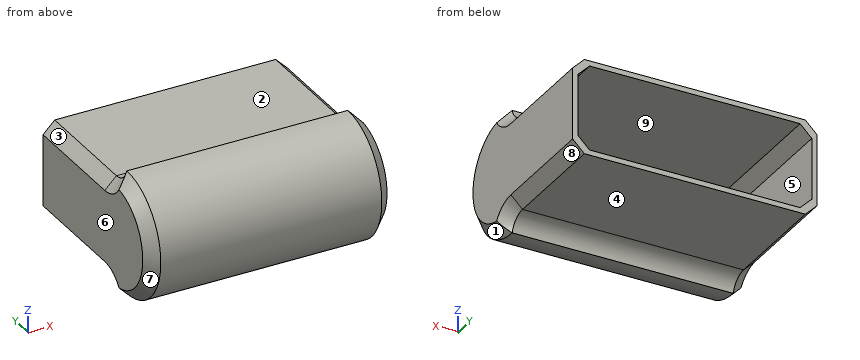
from build123d import *

# Parameters (mm, degrees)
F4_DEPTH      = 0.8
F4_DEPTH_BACK = 36.9
F5_DEPTH      = 36.1
F6_T1_DEPTH   = 37.7
F7_SIZE       = 1.8
F8_SIZE       = 1.8


# Not quite as in the source:
# - a fillet or chamfer that OpenCascade refuses, or shapes differently, is made with other operations: its cross-section is extruded or revolved along the edge and cut away or added


with BuildPart() as f4:
    # F3 (on Right) → F4 (new body, two sides)
    with BuildSketch(Plane.YZ) as f4_sk:
        with BuildLine():
            Line((20.2, 6.5358882766), (0, 6.5358882766))
            ThreePointArc((0, 6.5358882766), (-6.5358882766, 0), (0, -6.5358882766))
            Line((0, -6.5358882766), (20.2, -6.5358882766))
            Line((20.2, -6.5358882766), (20.2, 6.5358882766))
        make_face()
        with BuildLine():
            ThreePointArc((0, -6.5358882766), (-6.5358882766, 0), (0, 6.5358882766))
            Line((0, 6.5358882766), (20.2, 6.5358882766))
            Line((20.2, 6.5358882766), (20.2, 7.3358882766))
            Line((20.2, 7.3358882766), (0, 7.3358882766))
            Line((0, 7.3358882766), (0, 9.5358882766))
            ThreePointArc((0, 9.5358882766), (-9.5358882766, 0), (0, -9.5358882766))
            Line((0, -9.5358882766), (0, -7.3358882766))
            Line((0, -7.3358882766), (20.2, -7.3358882766))
            Line((20.2, -7.3358882766), (20.2, -6.5358882766))
            Line((20.2, -6.5358882766), (0, -6.5358882766))
        make_face()
    extrude(amount=-F4_DEPTH)
    extrude(f4_sk.sketch, amount=F4_DEPTH_BACK)

    # F3 (on Right) → F5 (cut)
    with BuildSketch(Plane.YZ):
        with BuildLine():
            Line((20.2, 6.5358882766), (0, 6.5358882766))
            ThreePointArc((0, 6.5358882766), (-6.5358882766, 0), (0, -6.5358882766))
            Line((0, -6.5358882766), (20.2, -6.5358882766))
            Line((20.2, -6.5358882766), (20.2, 6.5358882766))
        make_face()
    extrude(amount=F5_DEPTH, mode=Mode.SUBTRACT)

    # F6: fillet of radius 3 on 2 edges, made by hand

    # F6_s2 → F6_t1 (join)
    with BuildSketch(Plane.YZ.offset(-0.8)):
        with BuildLine():
            ThreePointArc((2.891366459, 7.3358882766), (1.0747762465, 7.9484209993), (0, 9.5358882766))
            Line((0, 9.5358882766), (0, 7.3358882766))
            Line((0, 7.3358882766), (2.891366459, 7.3358882766))
        make_face()
        with BuildLine():
            ThreePointArc((0, -9.5358882766), (1.0747762465, -7.9484209993), (2.891366459, -7.3358882766))
            Line((2.891366459, -7.3358882766), (0, -7.3358882766))
            Line((0, -7.3358882766), (0, -9.5358882766))
        make_face()
    extrude(amount=F6_T1_DEPTH)

    # F7
    f7_edges = [f4.edges().sort_by_distance(p)[0] for p in [
        (36.1, 10.1, 6.535888),
        (0, -6.535888, 0),
    ]]
    chamfer(f7_edges, length=F7_SIZE)

    # F8
    f8_edges = [f4.edges().sort_by_distance(p)[0] for p in [
        (36.9, 11.545683, 7.335888),
        (36.9, 1.074776, 7.948421),
        (36.9, -9.535888, 0),
        (36.9, 1.074776, -7.948421),
        (36.9, 11.545683, -7.335888),
        (-0.8, 11.545683, 7.335888),
        (-0.8, 1.074776, 7.948421),
        (-0.8, -9.535888, 0),
        (-0.8, 1.074776, -7.948421),
        (-0.8, 11.545683, -7.335888),
    ]]
    chamfer(f8_edges, length=F8_SIZE)


solid = f4.part
Geometry: final body of the model. Coordinates: model frame, mm. Face numbers are marked on the shaded views. A direction names the side the tool comes from. Give positions to 0.01 mm unless a question says otherwise; leave off trailing zeros. Write each loop counter-clockwise with the first axis right and the second up, starting at its lowest first coordinate (ties: lowest second). Pieces come first, ordered by that corner, then holes. Notation, with made-up numbers: M 80.25,67 L 120.25,67 A12 cw 120.25,72 Z; hole C 3,22 d5. An arc over 180 degrees is marked long. Answer in a Markdown table with one row per item. Add a question column.
(1) Section A-A on y = 14. Return loops of the section in (x, z), and give its area (3 significant figures).
(2) Reachability of the marked faces 1, 2, 3, 4 and 5 from +Z, -Z, +X, -X, +Y, -Y: full face, straight path, thin tool, end or side. Return the list, or none.
(3) Mould query, pull axis Z, two halves, no side actions, for the marked faces 6, 7, 8 and 9. Classes: +Z half, -Z half, draft (parallel to the pull), parting line (faces both ways), or undercut.
(4) First-contact query: pin 1 (10 mm diameter, centred on x = 25, y = 5.5, fed in from -Z); pin 2 (1 mm diameter, centred on y = 4, z = -6, fed in from -X); pin 3 (1.5 mm diameter, centred on x = 30, y = 12.5, fed in from +Z); pin 4 (1 mm diameter, centred on x = 14, z = -2.5, fed in from -Y). Flat tips, straight axial feed; report the tip coordinate or a pass-through.
(5) Section C-C on z = 0. Return loops of the section in (x, y).
(6) Section B-B on x = 15. Return loops of the section in (y, z), and give its area (3 significant figures).
(7) Ray query, line 1 (Z direction, x = 26, y = 4.5); line 2 (X direction, y = -3, z = 2); line 3 (X direction, y = 16.5, z = -6.25). Return the intervals inside material, ascending.
Result set:
| question | item | result |
|---|---|---|
| 1 | outline | M -0.8,-5.54 L 1,-7.34 L 35.1,-7.34 L 36.9,-5.54 L 36.9,5.54 L 35.1,7.34 L 1,7.34 L -0.8,5.54 Z; hole M 0,-4.74 L 1.8,-6.54 L 34.3,-6.54 L 36.1,-4.74 L 36.1,4.74 L 34.3,6.54 L 1.8,6.54 L 0,4.74 Z |
| 1 | area | 81.2 mm^2 |
| 2 | face 1 | +X, -Y |
| 2 | face 2 | +Z, +X, -X, +Y |
| 2 | face 3 | +Z, -X, +Y |
| 2 | face 4 | -Z, +X, -X, +Y |
| 2 | face 5 | +Y |
| 3 | face 6 | draft |
| 3 | face 7 | parting line |
| 3 | face 8 | -Z half |
| 3 | face 9 | undercut |
| 4 | pin 1 | stops at z = -8.52 |
| 4 | pin 2 | stops at x = -0.8 |
| 4 | pin 3 | stops at z = 7.34 |
| 4 | pin 4 | stops at y = -9.32 |
| 5 | outline | M -0.8,-7.74 L 1,-9.54 L 35.1,-9.54 L 36.9,-7.74 L 36.9,20.2 L 36.1,20.2 L 36.1,-4.74 L 34.3,-6.54 L 1.8,-6.54 L 0,-4.74 L 0,20.2 L -0.8,20.2 Z |
| 6 | outline | M 0,-9.54 A3 cw 2.89,-7.34 L 20.2,-7.34 L 20.2,-6.54 L 0,-6.54 A6.54 cw 0,6.54 L 20.2,6.54 L 20.2,7.34 L 2.89,7.34 A3 cw 0,9.54 A9.54 ccw Z |
| 6 | area | 111 mm^2 |
| 7 | line 1 | z = -7.34 to -6.54, 6.54 to 7.34 |
| 7 | line 2 | x = -0.8 to 0, 36.1 to 36.9 |
| 7 | line 3 | x = -0.09 to 1.51, 34.59 to 36.19 |
